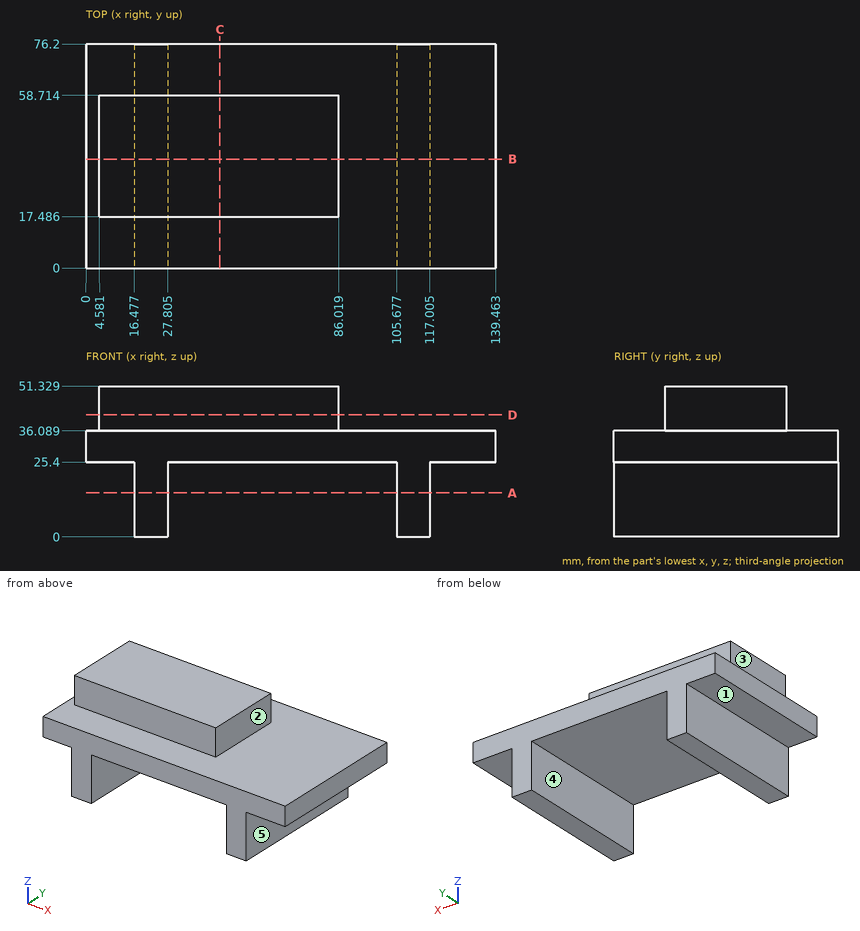
Drawing for the job (mm, zero at the part's lowest x, y, z). A direction names the side the tool comes from. Round coordinates to 2 decimals unless told otherwise and drop trailing zeros. Loops run counter-clockwise (first coordinate to the right, second up) from the corner with the lowest first, then second, coordinate; pieces in that order, holes last. Notation, with made-up numbers: (86.25, -34.75) -> (140.25, -34.75) arc R17 ccw to (140.25, -22.75) -> close; hole circle Ø7 at (-16, -40). An arc over 180 degrees is marked (long way). Use one line per item in the form item = value. Start each with the question number.
Item 1: Drop flat-ended pins along their axis: pin 1 Ø4.5 at (y, z) = (43.5, 41.5) entering from +X; pin 2 Ø5 at (x, y) = (10.5, 24.5) entering from -Z; pin 3 Ø7.5 at (y, z) = (52.5, 12.5) entering from -X. Give the stop position or say it passes through.
Item 2: Band-saw the part on B-B (y = 37). List the corners of the cut face in (x, z) (1 decimal), plus the area to 3 significant figures.
Item 3: Tool access for the marked faces 1, 2, 3, 4 and 5: list every direction of +Z, -Z, +X, -X, +Y, -Y with a clear straight run to the whole face (end or side of a thin tool).
Item 4: Band-saw the part on C-C (x = 45.5). List the corners of the cut face in (y, z), plus the area to 3 significant figures.
Item 5: Drill centre lines: line 1 along X through (y, z) = (10, 17) (1 decimal); line 2 along Z through (x, y) = (68, 39.5); line 3 along Z through (x, y) = (45.5, 62.5). Where is each one in solid material? Low to high.
Item 6: Band-saw the part on A-A (z = 15). List the corners of the cut face in (x, y) (1 decimal).
Item 7: Band-saw the part on D-D (z = 41.5). List the corners of the cut face in (x, y), plus the area to 3 significant figures.
Data:
q1.pin_1 = 86.02
q1.pin_2 = 25.4
q1.pin_3 = 16.48
q2.outline = (0, 25.4) -> (16.5, 25.4) -> (16.5, 0) -> (27.8, 0) -> (27.8, 25.4) -> (105.7, 25.4) -> (105.7, 0) -> (117, 0) -> (117, 25.4) -> (139.5, 25.4) -> (139.5, 36.1) -> (86, 36.1) -> (86, 51.3) -> (4.6, 51.3) -> (4.6, 36.1) -> (0, 36.1) -> close
q2.area = 3,310 mm^2
q3.face_1 = -Z, -X, +Y, -Y
q3.face_2 = +Z, +X, +Y, -Y
q3.face_3 = +Z, -X, +Y, -Y
q3.face_4 = -Z, +Y, -Y
q3.face_5 = -Z, +X, +Y, -Y
q4.outline = (0, 25.4) -> (76.2, 25.4) -> (76.2, 36.09) -> (58.71, 36.09) -> (58.71, 51.33) -> (17.49, 51.33) -> (17.49, 36.09) -> (0, 36.09) -> close
q4.area = 1,440 mm^2
q5.line_1 = 16.5 to 27.8, 105.7 to 117
q5.line_2 = 25.4 to 51.33
q5.line_3 = 25.4 to 36.09
q6.outline = (16.5, 0) -> (27.8, 0) -> (27.8, 76.2) -> (16.5, 76.2) -> close; (105.7, 0) -> (117, 0) -> (117, 76.2) -> (105.7, 76.2) -> close
q7.outline = (4.58, 17.49) -> (86.02, 17.49) -> (86.02, 58.71) -> (4.58, 58.71) -> close
q7.area = 3,360 mm^2
